For this review, take the finished solid that the model builds, in its own axes (mm). A direction names the side the tool comes from. Give positions to 0.01 mm unless a question says otherwise; leave off trailing zeros. Write each loop counter-clockwise with the first axis right and the second up, starting at its lowest first coordinate (ties: lowest second). Pieces come first, ordered by that corner, then holes. Notation, with made-up numbers: (79.5, 73) -> (115.5, 73) arc R29 cw to (115.5, 102) -> close; hole circle Ø8 at (15, -14.75). An arc over 180 degrees is marked (long way). Answer as CSV lines item,"result".
```python
from build123d import *

# Parameters (mm, degrees)
SKETCH1_R           = 1.65
SKETCH1_W           = 16
SKETCH1_H           = 3
BOSS_EXTRUDE1_DEPTH = 3


with BuildPart() as part:
    # Sketch1 → Boss-Extrude1 (new body)
    with BuildSketch(Plane(origin=(0, 0, 0), x_dir=(1, 0, 0), z_dir=(0, 1, 0))):
        with BuildLine():
            Line((30, -12.5), (-30, -12.5))
            ThreePointArc((-30, -12.5), (-37.071067812, -9.571067812), (-40, -2.5))
            Line((-40, -2.5), (-40, 12.5))
            Line((-40, 12.5), (-24, 12.5))
            Line((-24, 12.5), (-24, 9.5))
            Line((-24, 9.5), (-8, 9.5))
            Line((-8, 9.5), (-8, 12.5))
            Line((-8, 12.5), (8, 12.5))
            Line((8, 12.5), (8, 9.5))
            Line((8, 9.5), (24, 9.5))
            Line((24, 9.5), (24, 12.5))
            Line((24, 12.5), (40, 12.5))
            Line((40, 12.5), (40, -2.5))
            ThreePointArc((40, -2.5), (37.071067812, -9.571067812), (30, -12.5))
        make_face()
        with Locations((-15, -0.5)):
            Circle(SKETCH1_R, mode=Mode.SUBTRACT)
        with Locations((15, -0.5)):
            Circle(SKETCH1_R, mode=Mode.SUBTRACT)
        with Locations((-16, 5)):
            Rectangle(SKETCH1_W, SKETCH1_H, mode=Mode.SUBTRACT)
        with Locations((16, 5)):
            Rectangle(SKETCH1_W, SKETCH1_H, mode=Mode.SUBTRACT)
    extrude(amount=BOSS_EXTRUDE1_DEPTH)


solid = part.part
```
Q1. To check wall thickness, follow probe 1 along X at (y, z) = (1.3, 0.5); probe 2 along X at (y, z) = (0.9, -4.5); probe 3 along Z at (x, y) = (15, 2.25). State the ranges of each line that lie inside material, in increasing order. Write a range as [from, to].
Answer block:
probe 1,"x = [-40, -16.65], [-13.35, 13.35], [16.65, 40]"
probe 2,"x = [-40, -24], [-8, 8], [24, 40]"
probe 3,"z = [-9.5, -6.5], [-3.5, -1.15], [2.15, 12.5]"
Q2. Add section C-C (y = 1). Write out the cut boundary in (x, z), plus the area to 3 significant figures.
Answer block:
outline,"(-40, -12.5) -> (-24, -12.5) -> (-24, -9.5) -> (-8, -9.5) -> (-8, -12.5) -> (8, -12.5) -> (8, -9.5) -> (24, -9.5) -> (24, -12.5) -> (40, -12.5) -> (40, 2.5) arc R10 ccw to (30, 12.5) -> (-30, 12.5) arc R10 ccw to (-40, 2.5) -> close; hole (-24, -6.5) -> (-8, -6.5) -> (-8, -3.5) -> (-24, -3.5) -> close; hole circle Ø3.3 at (-15, 0.5); hole (8, -6.5) -> (24, -6.5) -> (24, -3.5) -> (8, -3.5) -> close; hole circle Ø3.3 at (15, 0.5)"
area,"1,750 mm2"
Q3. Add section A-A (z = 0.5). Write out the cut boundary in (x, y), plus the area to 3 significant figures.
Answer block:
outline,"(-40, 0) -> (-16.65, 0) -> (-16.65, 3) -> (-40, 3) -> close; (-13.35, 0) -> (13.35, 0) -> (13.35, 3) -> (-13.35, 3) -> close; (16.65, 0) -> (40, 0) -> (40, 3) -> (16.65, 3) -> close"
area,"220 mm2"
Q4. For faces 1 (the flat face through (-24, 1, -11)), 2 (the flat face through (1, 3, 0)), 3 (the flat face through (8, 1, -5)), list the 3-axis set-ups (+Z, -Z, +X, -X, +Y, -Y) from which the entire face can be reached by the end or side of a thin tool; tool diameter is ignored.
Answer block:
face 1,"-Z, +Y, -Y"
face 2,"+Z, -Z, +X, -X, +Y"
face 3,"+Y, -Y"
Q5. Clearance check with flat-ended pins moving along their axes: pin 1 (1 mm diameter, centred on x = -17, y = 0.5, fed in from -Z); pin 2 (1.5 mm diameter, centred on x = -18.5, z = 8.5, fed in from -Y); pin 3 (2 mm diameter, centred on x = -15, z = 0.5, fed in from +Y). State where each tip first meets the part, or that it passes through.
Answer block:
pin 1,"stops at z = -9.5"
pin 2,"stops at y = 0"
pin 3,"passes through"
Q6. Draft analysis for pull direction X (two halves, no side actions). For faces 4 (the flat face through (-16, 1, -3.5)), 5 (the flat face through (0, 1, 12.5)), 6 (the cylindrical face through (-36.99, 1.48, 9.65)), 7 (the flat face through (-16, 1, -9.5)), state which applies: released by +X, released by -X, zero draft, split by the parting line, or undercut.
Answer block:
face 4,"undercut"
face 5,"zero draft"
face 6,"released by -X"
face 7,"undercut"
Q7. Add section B-B (x = -15). Write out the cut boundary in (y, z).
Answer block:
outline,"(0, -9.5) -> (3, -9.5) -> (3, -6.5) -> (0, -6.5) -> close; (0, -3.5) -> (3, -3.5) -> (3, -1.15) -> (0, -1.15) -> close; (0, 2.15) -> (3, 2.15) -> (3, 12.5) -> (0, 12.5) -> close"
